```python
from build123d import *

# Parameters (mm, degrees)
SKETCH1_R           = 1
SKETCH1_R_2         = 7.5
BOSS_EXTRUDE1_DEPTH = 2


with BuildPart() as part:
    # Sketch1 → Boss-Extrude1 (new body)
    # profile 1 of 2: a face of its own
    with BuildSketch(Plane.XY):
        with BuildLine():
            ThreePointArc((-36.032258065, 10.893868862), (-43, 0), (-36.032258065, -10.893868862))
            Line((-36.032258065, -10.893868862), (-10.483870968, -22.695560128))
            ThreePointArc((-10.483870968, -22.695560128), (8.421796013, -23.538762752), (22.501635968, -10.893868862))
            ThreePointArc((22.501635968, -10.893868862), (25, 0), (22.501635968, 10.893868862))
            ThreePointArc((22.501635968, 10.893868862), (8.421796013, 23.538762752), (-10.483870968, 22.695560128))
            Line((-10.483870968, 22.695560128), (-36.032258065, 10.893868862))
        make_face()
        with Locations(Location((8.154330676, 12.589951995, 0), (0, 0, 180))):
            Circle(SKETCH1_R, mode=Mode.SUBTRACT)
        with Locations(Location((-8.154330676, -12.589951995, 0), (0, 0, 180))):
            Circle(SKETCH1_R, mode=Mode.SUBTRACT)
        with Locations((-31, 0)):
            Circle(SKETCH1_R_2, mode=Mode.SUBTRACT)
        with Locations(Location((12.589951995, -8.154330676, 0), (0, 0, 180))):
            Circle(SKETCH1_R, mode=Mode.SUBTRACT)
        with Locations(Location((-12.589951995, 8.154330676, 0), (0, 0, 180))):
            Circle(SKETCH1_R, mode=Mode.SUBTRACT)
    # profile 2 of 2: a face of its own
    with BuildSketch(Plane.XY):
        with Locations((-31, 0)):
            Circle(SKETCH1_R_2)
        with BuildLine():
            ThreePointArc((-35.198052011, 1.620604614), (-29.379395386, 4.198052011), (-26.801947989, -1.620604614))
            ThreePointArc((-26.801947989, -1.620604614), (-32.620604614, -4.198052011), (-35.198052011, 1.620604614))
        make_face(mode=Mode.SUBTRACT)
    extrude(amount=BOSS_EXTRUDE1_DEPTH)


solid = part.part
```
Build history of the part. All positions in model axes, mm. Give positions to 0.01 mm unless a question says otherwise; leave off trailing zeros. Loops run counter-clockwise (first coordinate to the right, second up) from the corner with the lowest first, then second, coordinate; pieces in that order, holes last. Notation, with made-up numbers: (62, 69.25) - (80, 69.25) arc R21 ccw to (80, 107.25) - close; hole circle Ø4 at (52, -30.5). An arc over 180 degrees is marked (long way). Use a Markdown table: item, result.
(1) Band-saw the part on C-C (z = 0.4). Give the cut face in (x, y), and give its area (3 significant figures).
Taken from the geometry:
| item | result |
|---|---|
| outline | (-36.03, -10.89) - (-10.48, -22.7) arc R25 ccw (long way) to (-10.48, 22.7) - (-36.03, 10.89) arc R12 ccw to start; hole circle Ø9 at (-31, 0); hole circle Ø2 at (-12.59, 8.15); hole circle Ø2 at (-8.15, -12.59); hole circle Ø2 at (8.15, 12.59); hole circle Ø2 at (12.59, -8.15) |
| area | 2,380 mm2 |
(2) Band-saw the part on D-D (x = -38.5). Give the cut face in (y, z), and give its area (3 significant figures).
Taken from the geometry:
| item | result |
|---|---|
| outline | (-9.37, 0) - (9.37, 0) - (9.37, 2) - (-9.37, 2) - close |
| area | 37.5 mm2 |
(3) Band-saw the part on B-B (x = -31). Give the cut face in (y, z), and give its area (3 significant figures).
Taken from the geometry:
| item | result |
|---|---|
| outline | (-13.22, 0) - (-4.5, 0) - (-4.5, 2) - (-13.22, 2) - close; (4.5, 0) - (13.22, 0) - (13.22, 2) - (4.5, 2) - close |
| area | 34.9 mm2 |
(4) Wall check: line 1 along X through (y, z) = (0, 1.15); line 2 along Y through (x, z) = (-28, 0.7); line 3 along Y through (x, z) = (-31, 1.85). Give the ranges that are in metal, low to high.
Taken from the geometry:
| item | result |
|---|---|
| line 1 | -43 to -35.5, -26.5 to 25 |
| line 2 | -14.6 to -3.35, 3.35 to 14.6 |
| line 3 | -13.22 to -4.5, 4.5 to 13.22 |
(5) Pull direction X, two halves, no side cores. Call faces 1 (the face through (-9, 0, 2)), 2 (the face through (-43, 0, 1)), 3 (the face through (-11.59, 8.11, 0.99)): +X half, -X half, draft (parallel to the pull), parting line (faces both ways), or undercut.
Taken from the geometry:
| item | result |
|---|---|
| face 1 | draft |
| face 2 | -X half |
| face 3 | undercut |
(6) Drop a flat-ended pin along its axis: pin 1 Ø1 at (y, z) = (-1.5, 1) entering from -X. Give the stop position or say it passes through.
Taken from the geometry:
| item | result |
|---|---|
| pin 1 | x = -42.96 |
(7) Band-saw the part on A-A (y = 0). Give the cut face in (x, z), and give its area (3 significant figures).
Taken from the geometry:
| item | result |
|---|---|
| outline | (-43, 0) - (-35.5, 0) - (-35.5, 2) - (-43, 2) - close; (-26.5, 0) - (25, 0) - (25, 2) - (-26.5, 2) - close |
| area | 118 mm2 |
